Part model, mm, in its own coordinate system. Face numbers are marked on the shaded views. A direction names the side the tool comes from. Give positions to 0.01 mm unless a question says otherwise; leave off trailing zeros. Write each loop counter-clockwise with the first axis right and the second up, starting at its lowest first coordinate (ties: lowest second). Pieces come first, ordered by that corner, then holes.
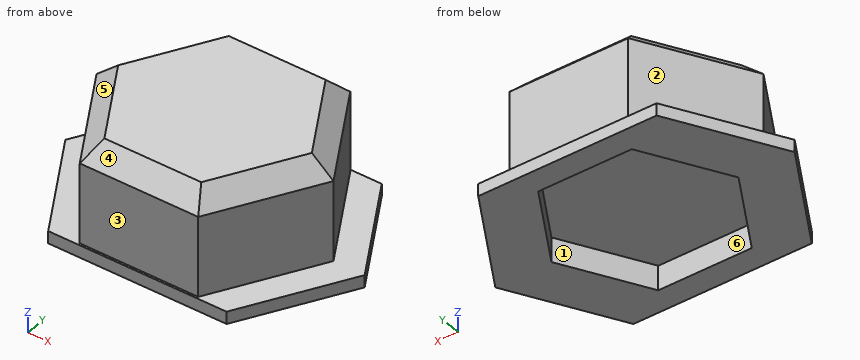
from build123d import *

# Parameters (mm, degrees)
BOX036_W        = 26
BOX036_H        = 10
BOX036_DEPTH    = 10
BOX035_W        = 26
BOX035_H        = 10
BOX035_DEPTH    = 10
PRISM011_DEPTH  = 2
PRISM010_DEPTH  = 1
PRISM009_DEPTH  = 9
CHAMFER006_SIZE = 1.5


with BuildPart() as cubo032:
    # Box036 → Box036 (new body)
    with BuildSketch(Plane(origin=(-95, -18.4, 0), x_dir=(1, 0, 0), z_dir=(0, 0, 1))):
        with Locations((13, 5)):
            Rectangle(BOX036_W, BOX036_H)
    extrude(amount=BOX036_DEPTH)


with BuildPart() as fusion016:
    # Box035 → Box035 (new body)
    with BuildSketch(Plane(origin=(-95, 8.4, 0), x_dir=(1, 0, 0), z_dir=(0, 0, 1))):
        with Locations((13, 5)):
            Rectangle(BOX035_W, BOX035_H)
    extrude(amount=BOX035_DEPTH)

    # Fusion016: union Cubo032
    add(cubo032.part)


with BuildPart() as prisma008:
    # Prism011 → Prism011 (new body)
    with BuildSketch(Plane.XY):
        Polygon((7.5, 0), (3.75, 6.495191), (-3.75, 6.495191), (-7.5, 0), (-3.75, -6.495191), (3.75, -6.495191), align=None)
    extrude(amount=PRISM011_DEPTH)


with BuildPart() as prisma007:
    # Prism010 → Prism010 (new body)
    with BuildSketch(Plane.XY):
        Polygon((12, 0), (6, 10.392305), (-6, 10.392305), (-12, 0), (-6, -10.392305), (6, -10.392305), align=None)
    extrude(amount=PRISM010_DEPTH)


with BuildPart() as chamfer006:
    # Prism009 → Prism009 (new body)
    with BuildSketch(Plane.XY):
        Polygon((9.5, 0), (4.75, 8.227241), (-4.75, 8.227241), (-9.5, 0), (-4.75, -8.227241), (4.75, -8.227241), align=None)
    extrude(amount=PRISM009_DEPTH)

    # Fusion015: union Prisma007
    add(prisma007.part)

    # Cut018: cut Prisma008
    add(prisma008.part, mode=Mode.SUBTRACT)


with BuildPart() as chamfer006_1:
    # Cut018 placement: moved
    add(chamfer006.part.moved(Location((-81, 0, 0))))

    # Cut019: cut Fusion016
    add(fusion016.part, mode=Mode.SUBTRACT)

    # Chamfer006
    chamfer006_edges = [chamfer006_1.edges().sort_by_distance(p)[0] for p in [
        (-73.875, 4.113621, 9),
        (-73.875, -4.113621, 9),
        (-81, 8.227241, 9),
        (-81, -8.227241, 9),
        (-88.125, 4.113621, 9),
        (-88.125, -4.113621, 9),
    ]]
    chamfer(chamfer006_edges, length=CHAMFER006_SIZE)


solid = chamfer006_1.part
1) Saw through at B-B (x = -81.75). Write the cut outline in (y, z), and give its area (3 significant figures).
Check result:
outline: (-8.4, 0) - (-6.5, 0) - (-6.5, 2) - (6.5, 2) - (6.5, 0) - (8.4, 0) - (8.4, 1) - (8.23, 1) - (8.23, 7.5) - (6.73, 9) - (-6.73, 9) - (-8.23, 7.5) - (-8.23, 1) - (-8.4, 1) - close
area: 120 mm2
2) Saw through at D-D (z = 8.25). Write the cut outline in (x, y), and give its area (3 significant figures).
Check result:
outline: (-89.63, 0) - (-85.32, -7.48) - (-76.68, -7.48) - (-72.37, 0) - (-76.68, 7.48) - (-85.32, 7.48) - close
area: 194 mm2
3) Saw through at A-A (y = -4.25). Write the cut outline in (x, z), and give its area (3 significant figures).
Check result:
outline: (-90.55, 0) - (-86.05, 0) - (-86.05, 2) - (-75.95, 2) - (-75.95, 0) - (-71.45, 0) - (-71.45, 1) - (-73.95, 1) - (-73.95, 7.5) - (-75.69, 9) - (-86.31, 9) - (-88.05, 7.5) - (-88.05, 1) - (-90.55, 1) - close
area: 109 mm2
4) Drill centre lines: L1, parallel to Y at x = -80.75, z = 1.5; L2, parallel to Z at x = -72.5, y = 3.75; L3, parallel to X at y = -6.25, z = 1.75. Where is each one in solid material? Low to high.
Check result:
L1: y = -8.23 to -6.5, 6.5 to 8.23
L2: z = 0 to 1
L3: x = -86.89 to -84.89, -77.11 to -75.11
5) Flat gauge pins, fed straight in: P1, Ø1.5, axis at y = -1, z = 5, coming from the +X side; P2, Ø2, axis at x = -81, z = 4.5, coming from the +Y side; P3, Ø1, axis at x = -79, z = 6.5, coming from the -Y side. Where does each tip first touch, or does it go through?
Check result:
P1: stops at x = -71.64
P2: stops at y = 8.23
P3: stops at y = -8.23
6) Saw through at C-C (z = 6.25). Write the cut outline in (x, y).
Check result:
outline: (-90.5, 0) - (-85.75, -8.23) - (-76.25, -8.23) - (-71.5, 0) - (-76.25, 8.23) - (-85.75, 8.23) - close
7) Mould opens along X. For the marked faces 4, 5 and 6 say: +X half, -X half, draft (parallel to the pull), parting line (faces both ways), or undercut.
Check result:
face 4: draft
face 5: -X half
face 6: undercut
8) 3-axis set-ups, long thin cutter, end or side, ignore diameter. For the marked faces 1, 2 and 3: which of +Z, -Z, +X, -X, +Y, -Y reach the whole face in a straight line?
Check result:
face 1: -Z
face 2: +Z, -X, +Y
face 3: +Z, +X, -X, -Y
